from build123d import *

# Parameters (mm, degrees)
F0_W      = 130
F0_H      = 75
F1_DEPTH  = 12
F3_DEPTH  = 345
F5_D      = 12
F7_DEPTH  = 50.8
F8_W      = 70
F8_H      = 130
F9_DEPTH  = 12
F11_D     = 5
F11_DEPTH = 8
F11_TIP   = 1.5021515476


with BuildPart() as f1:
    # F0 (on Top) → F1 (new body)
    with BuildSketch(Plane.XY):
        Rectangle(F0_W, F0_H)
    extrude(amount=-F1_DEPTH)

    # F2 (on face) → F3 (join)
    with BuildSketch(Plane.XY):
        with BuildLine():
            Line((-19.05, -25.4), (19.05, -25.4))
            ThreePointArc((19.05, -25.4), (23.5401280605, -23.5401280605), (25.4, -19.05))
            Line((25.4, -19.05), (25.4, 19.05))
            ThreePointArc((25.4, 19.05), (23.5401280605, 23.5401280605), (19.05, 25.4))
            Line((19.05, 25.4), (-19.05, 25.4))
            ThreePointArc((-19.05, 25.4), (-23.5401280605, 23.5401280605), (-25.4, 19.05))
            Line((-25.4, 19.05), (-25.4, -19.05))
            ThreePointArc((-25.4, -19.05), (-23.5401280605, -23.5401280605), (-19.05, -25.4))
        make_face()
        with BuildLine():
            Line((-12.7, 19.05), (12.7, 19.05))
            ThreePointArc((12.7, 19.05), (17.1901280605, 17.1901280605), (19.05, 12.7))
            Line((19.05, 12.7), (19.05, -12.7))
            ThreePointArc((19.05, -12.7), (17.1901280605, -17.1901280605), (12.7, -19.05))
            Line((12.7, -19.05), (-12.7, -19.05))
            ThreePointArc((-12.7, -19.05), (-17.1901280605, -17.1901280605), (-19.05, -12.7))
            Line((-19.05, -12.7), (-19.05, 12.7))
            ThreePointArc((-19.05, 12.7), (-17.1901280605, 17.1901280605), (-12.7, 19.05))
        make_face(mode=Mode.SUBTRACT)
    extrude(amount=F3_DEPTH)

    # F5 (through all)
    with Locations(Plane.XY):
        with Locations((-53, 22.5), (53, 22.5), (53, -22.5), (-53, -22.5)):
            Hole(F5_D / 2)

    # F6 (on face) → F7 (cut)
    with BuildSketch(Plane.YZ.offset(25.4)):
        Polygon((-19.05, 345), (-25.4, 345), (-25.4, 244.9542985566), (-19.05, 257.460011237), align=None)
        Polygon((19.05, 345), (-19.05, 345), (-19.05, 257.460011237), (19.05, 332.4942873196), align=None)
        Polygon((25.4, 345), (19.05, 345), (19.05, 332.4942873196), align=None)
    extrude(amount=-F7_DEPTH, mode=Mode.SUBTRACT)

    # F8 (on face) → F9 (join)
    with BuildSketch(Plane(origin=(0, -119.0782097883, 60.4640976071), x_dir=(1, 0, 0), z_dir=(0, -0.8916395458, 0.4527459778))):
        with Locations((0, 263.0132913952)):
            Rectangle(F8_W, F8_H)
        with BuildLine():
            Line((25.4, 305.0898661941), (25.4, 220.9367165963))
            add(Edge.make_bspline(
                [(25.4, 220.9367165963), (25.4, 206.9111916633), (19.05, 206.9111916633)],
                knots=[4.7123889804, 4.7123889804, 4.7123889804, 6.2831853072, 6.2831853072, 6.2831853072], degree=2, weights=[1, 0.7071067812, 1]))
            Line((19.05, 206.9111916633), (-19.05, 206.9111916633))
            add(Edge.make_bspline(
                [(-19.05, 206.9111916633), (-25.4, 206.9111916633), (-25.4, 220.9367165963)],
                knots=[0, 0, 0, 1.5707963268, 1.5707963268, 1.5707963268], degree=2, weights=[1, 0.7071067812, 1]))
            Line((-25.4, 220.9367165963), (-25.4, 305.0898661941))
            add(Edge.make_bspline(
                [(-25.4, 305.0898661941), (-25.4, 319.115391127), (-19.05, 319.115391127)],
                knots=[1.5707963268, 1.5707963268, 1.5707963268, 3.1415926536, 3.1415926536, 3.1415926536], degree=2, weights=[1, 0.7071067812, 1]))
            Line((-19.05, 319.115391127), (19.05, 319.115391127))
            add(Edge.make_bspline(
                [(19.05, 319.115391127), (25.4, 319.115391127), (25.4, 305.0898661941)],
                knots=[3.1415926536, 3.1415926536, 3.1415926536, 4.7123889804, 4.7123889804, 4.7123889804], degree=2, weights=[1, 0.7071067812, 1]))
        make_face(mode=Mode.SUBTRACT)
        with BuildLine():
            add(Edge.make_bspline(
                [(25.4, 220.9367165963), (25.4, 206.9111916633), (19.05, 206.9111916633)],
                knots=[4.7123889804, 4.7123889804, 4.7123889804, 6.2831853072, 6.2831853072, 6.2831853072], degree=2, weights=[1, 0.7071067812, 1]))
            Line((25.4, 220.9367165963), (25.4, 305.0898661941))
            add(Edge.make_bspline(
                [(19.05, 319.115391127), (25.4, 319.115391127), (25.4, 305.0898661941)],
                knots=[3.1415926536, 3.1415926536, 3.1415926536, 4.7123889804, 4.7123889804, 4.7123889804], degree=2, weights=[1, 0.7071067812, 1]))
            Line((19.05, 319.115391127), (-19.05, 319.115391127))
            add(Edge.make_bspline(
                [(-25.4, 305.0898661941), (-25.4, 319.115391127), (-19.05, 319.115391127)],
                knots=[1.5707963268, 1.5707963268, 1.5707963268, 3.1415926536, 3.1415926536, 3.1415926536], degree=2, weights=[1, 0.7071067812, 1]))
            Line((-25.4, 305.0898661941), (-25.4, 220.9367165963))
            add(Edge.make_bspline(
                [(-19.05, 206.9111916633), (-25.4, 206.9111916633), (-25.4, 220.9367165963)],
                knots=[0, 0, 0, 1.5707963268, 1.5707963268, 1.5707963268], degree=2, weights=[1, 0.7071067812, 1]))
            Line((-19.05, 206.9111916633), (19.05, 206.9111916633))
        make_face()
        with BuildLine():
            Line((-19.05, 234.9622415292), (-19.05, 291.0643412611))
            add(Edge.make_bspline(
                [(-19.05, 291.0643412611), (-19.05, 305.0898661941), (-12.7, 305.0898661941)],
                knots=[1.5707963268, 1.5707963268, 1.5707963268, 3.1415926536, 3.1415926536, 3.1415926536], degree=2, weights=[1, 0.7071067812, 1]))
            Line((-12.7, 305.0898661941), (12.7, 305.0898661941))
            add(Edge.make_bspline(
                [(12.7, 305.0898661941), (19.05, 305.0898661941), (19.05, 291.0643412611)],
                knots=[3.1415926536, 3.1415926536, 3.1415926536, 4.7123889804, 4.7123889804, 4.7123889804], degree=2, weights=[1, 0.7071067812, 1]))
            Line((19.05, 291.0643412611), (19.05, 234.9622415292))
            add(Edge.make_bspline(
                [(19.05, 234.9622415292), (19.05, 220.9367165963), (12.7, 220.9367165963)],
                knots=[4.7123889804, 4.7123889804, 4.7123889804, 6.2831853072, 6.2831853072, 6.2831853072], degree=2, weights=[1, 0.7071067812, 1]))
            Line((12.7, 220.9367165963), (-12.7, 220.9367165963))
            add(Edge.make_bspline(
                [(-12.7, 220.9367165963), (-19.05, 220.9367165963), (-19.05, 234.9622415292)],
                knots=[0, 0, 0, 1.5707963268, 1.5707963268, 1.5707963268], degree=2, weights=[1, 0.7071067812, 1]))
        make_face(mode=Mode.SUBTRACT)
        with BuildLine():
            add(Edge.make_bspline(
                [(-19.05, 291.0643412611), (-19.05, 305.0898661941), (-12.7, 305.0898661941)],
                knots=[1.5707963268, 1.5707963268, 1.5707963268, 3.1415926536, 3.1415926536, 3.1415926536], degree=2, weights=[1, 0.7071067812, 1]))
            Line((-19.05, 291.0643412611), (-19.05, 234.9622415292))
            add(Edge.make_bspline(
                [(-12.7, 220.9367165963), (-19.05, 220.9367165963), (-19.05, 234.9622415292)],
                knots=[0, 0, 0, 1.5707963268, 1.5707963268, 1.5707963268], degree=2, weights=[1, 0.7071067812, 1]))
            Line((-12.7, 220.9367165963), (12.7, 220.9367165963))
            add(Edge.make_bspline(
                [(19.05, 234.9622415292), (19.05, 220.9367165963), (12.7, 220.9367165963)],
                knots=[4.7123889804, 4.7123889804, 4.7123889804, 6.2831853072, 6.2831853072, 6.2831853072], degree=2, weights=[1, 0.7071067812, 1]))
            Line((19.05, 234.9622415292), (19.05, 291.0643412611))
            add(Edge.make_bspline(
                [(12.7, 305.0898661941), (19.05, 305.0898661941), (19.05, 291.0643412611)],
                knots=[3.1415926536, 3.1415926536, 3.1415926536, 4.7123889804, 4.7123889804, 4.7123889804], degree=2, weights=[1, 0.7071067812, 1]))
            Line((12.7, 305.0898661941), (-12.7, 305.0898661941))
        make_face()
    extrude(amount=F9_DEPTH)

    # F11
    with Locations(Plane(origin=(0, -129.7778843376, 65.8970493408), x_dir=(1, 0, 0), z_dir=(0, -0.8916395458, 0.4527459778))):
        with Locations((15, 298.0132913952), (15, 253.0132913952), (-15, 253.0132913952), (-15, 298.0132913952)):
            Hole(F11_D / 2, depth=F11_DEPTH)
            with Locations((0, 0, -(F11_DEPTH + F11_TIP / 2))):  # 118° drill point
                Cone(0, F11_D / 2, F11_TIP, mode=Mode.SUBTRACT)


solid = f1.part
Geometry check sheet. Reference: the model listing, model coordinates, mm. A direction names the side the tool comes from. Give positions to 0.01 mm unless a question says otherwise; leave off trailing zeros. Write each loop counter-clockwise with the first axis right and the second up, starting at its lowest first coordinate (ties: lowest second). Pieces come first, ordered by that corner, then holes. Notation, with made-up numbers: (48.25, 68) - (101.25, 68) arc R33 cw to (101.25, 102) - close; hole circle Ø8 at (51, 18.5). An arc over 180 degrees is marked (long way). Put each result on its own line as item: value.
1. Sectioned sample at A-A, the plane z = 151.5. Enter the section's corners in (x, y).
Ans:
outline: (-25.4, -19.05) arc R6.35 ccw to (-19.05, -25.4) - (19.05, -25.4) arc R6.35 ccw to (25.4, -19.05) - (25.4, 19.05) arc R6.35 ccw to (19.05, 25.4) - (-19.05, 25.4) arc R6.35 ccw to (-25.4, 19.05) - close; hole (-19.05, -12.7) arc R6.35 ccw to (-12.7, -19.05) - (12.7, -19.05) arc R6.35 ccw to (19.05, -12.7) - (19.05, 12.7) arc R6.35 ccw to (12.7, 19.05) - (-12.7, 19.05) arc R6.35 ccw to (-19.05, 12.7) - close
2. Sectioned sample at D-D, the plane x = 31.5. Enter the section's corners in (y, z).
Ans:
outline: (-40.13, 242.45) - (-29.43, 237.02) - (29.43, 352.93) - (18.73, 358.37) - close; (-37.5, -12) - (37.5, -12) - (37.5, 0) - (-37.5, 0) - close
3. Go/stop test with flat-tipped pins: pin 1 (11 mm diameter, centred on x = 53, y = 22.5, fed in from -Z); pin 2 (19 mm diameter, centred on x = 2, z = 144, fed in from +Y); pin 3 (7.5 mm diameter, centred on y = -0.5, z = 108, fed in from -X); pin 4 (8 mm diameter, centred on x = -3, z = 47.5, fed in from -Y). Record where each tip stops, or that it passes through.
Ans:
pin 1: passes through
pin 2: stops at y = 25.4
pin 3: stops at x = -25.4
pin 4: stops at y = -25.4
4. Draft check along Y on faces 1 (the flat face through (-65, -1, -6)), 2 (the flat face through (19.05, 0, 158)), 3 (the flat face through (-0.5, -10.3, 301.2)). Enter one of: +Y half, -Y half, draft (parallel to the pull), parting line (faces both ways), or undercut.
Ans:
face 1: draft
face 2: undercut
face 3: -Y half
5. Sectioned sample at C-C, the plane y = -34. Enter the section's corners in (x, z).
Ans:
outline: (-65, -12) - (65, -12) - (65, 0) - (-65, 0) - close; (-35, 239.34) - (35, 239.34) - (35, 254.52) - (-35, 254.52) - close
6. Thickness scan on line 1 (Y direction, x = 53, z = -7.5); line 2 (X direction, y = 22, z = -5); line 3 (X direction, y = -6.5, z = 40). Record the ranges inside material, lowest first.
Ans:
line 1: y = -37.5 to -28.5, -16.5 to 16.5, 28.5 to 37.5
line 2: x = -65 to -58.98, -47.02 to 47.02, 58.98 to 65
line 3: x = -25.4 to -19.05, 19.05 to 25.4
7. Sectioned sample at B-B, the plane x = 53. Enter the section's corners in (y, z).
Ans:
outline: (-37.5, -12) - (-28.5, -12) - (-28.5, 0) - (-37.5, 0) - close; (-16.5, -12) - (16.5, -12) - (16.5, 0) - (-16.5, 0) - close; (28.5, -12) - (37.5, -12) - (37.5, 0) - (28.5, 0) - close
8. Set-up check for faces 4 (the cylindrical face through (-23.49, 23.59, 170.08)), 5 (the flat face through (-31.601, 0.412, 295.789)), 6 (the flat face through (-35, -6, 297)): record each of +Z, -Z, +X, -X, +Y, -Y from which the full face is reachable in a straight line by a thin tool's end or side.
Ans:
face 4: -X, +Y
face 5: none
face 6: +Z, -X, +Y, -Y
